Check sheet for the modelled part. Datum: model origin and axes. Units: mm. A direction names the side the tool comes from. Round coordinates to 2 decimals unless told otherwise and drop trailing zeros. Return JSON: item names as keys, results as strings.
from build123d import *


with BuildPart() as f1:
    # F0 (on Front) → F1 (revolve)
    with BuildSketch(Plane.XZ):
        with BuildLine():
            Line((83.359114, -5.08), (83.359114, 0))
            Line((83.359114, 0), (45.259114, 0))
            Line((45.259114, 0), (45.259114, -24.796592))
            ThreePointArc((45.259114, -24.796592), (64.807486, -26.936857), (83.359114, -33.460405))
            Line((83.359114, -33.460405), (83.359114, -15.706522))
            Line((83.359114, -15.706522), (80.893344, -15.706522))
            Line((80.893344, -15.706522), (80.817882, -14.438765))
            Line((80.817882, -14.438765), (83.359114, -14.287501))
            Line((83.359114, -14.287501), (83.205484, -11.706533))
            Line((83.205484, -11.706533), (80.808878, -11.706533))
            Line((80.808878, -11.706533), (80.808878, -9.862984))
            Line((80.808878, -9.862984), (83.359114, -9.862984))
            Line((83.359114, -9.862984), (83.359114, -6.731))
            Line((83.359114, -6.731), (80.640316, -6.731))
            Line((80.640316, -6.731), (80.640316, -5.08))
            Line((80.640316, -5.08), (83.359114, -5.08))
        make_face()
    revolve(axis=Axis((45.259114, 0, -12.398296), (0, 0, -1)))


solid = f1.part
Q1. Material ranges on line 1 (X direction, y = -0.5, z = -14.5); line 2 (X direction, y = 1, z = -5); line 3 (Y direction, x = 73, z = -1.5), recorded low to high.
Results list:
{"line 1": "9.7 to 80.82", "line 2": "7.17 to 83.35", "line 3": "-26.12 to 26.12"}
Q2. Draft check along Z on faces 1 (the flat face through (45, -1, 0)), 2 (the flat face through (57, 34, -9.863)), 3 (the cylindrical face through (80.454, 14.593, -2.504)), 4 (the cylindrical face through (79.167, -10.678, -10.772)). Enter one of: released by +Z, released by -Z, zero draft, split by the parting line, or undercut.
Results list:
{"face 1": "released by +Z", "face 2": "undercut", "face 3": "zero draft", "face 4": "undercut"}
Q3. Tool access check on faces 5 (the cylindrical face through (80.454, 14.593, -24.459)), 6 (the flat face through (11, 11, -11.707)). Record the directions out of +Z, -Z, +X, -X, +Y, -Y that give a thin tool (end or side, any length) a straight path to the whole face; none if there is none.
Results list:
{"face 5": "+Z, -Z", "face 6": "none"}
Q4. Go/stop test with flat-tipped pins: pin 1 (10 mm diameter, centred on y = 27.5, z = -30, fed in from -X); pin 2 (3 mm diameter, centred on x = 66, y = -1, fed in from -Z); pin 3 (5 mm diameter, centred on x = 23, y = 3.5, fed in from -Z). Record where each tip stops, or that it passes through.
Results list:
{"pin 1": "x = 14.51", "pin 2": "z = -27.6", "pin 3": "z = -28.38"}
